Build history of the part. All positions in model axes, mm. A direction names the side the tool comes from. Round coordinates to 2 decimals unless told otherwise and drop trailing zeros. Order: outer loops, then holes, each group sorted by start corner. A loop starts at its lowest first (then second) coordinate and runs counter-clockwise, first axis right, second up. Notation, with made-up numbers: M 41,-39.5 L 72,-39.5 A33 cw 72,-2.5 Z; hole C -9,38 d7. An arc over 180 degrees is marked long. One line per item, written item: value. Start each with the question number.
Item 1: Band-saw the part on B-B, the plane x = 102. Write the cut outline in (y, z), then the cut area to 3 significant figures.
Item 2: Band-saw the part on A-A, the plane z = -15. Write the cut outline in (x, y), then the cut area to 3 significant figures.
Item 3: Band-saw the part on C-C, the plane y = 0.9. Give the number of separate pieces and of enclosed holes in the cut face, then the cut area to 3 significant figures.
Item 4: Probe L1, parallel to X at y = 2.6, z = -22.5; L2, parallel to Z at x = 81, y = 1.1; L3, parallel to X at y = 2.5, z = -5.5. List the from-to ranges inside material, lowest first.
Item 5: Band-saw the part on D-D, the plane x = 43.5. Write the cut outline in (y, z), then the cut area to 3 significant figures.
Item 6: Pin check, flat tip, straight feed: pin 1 (10 mm diameter, centred on x = -26.5, z = 28, fed in from -Y). Stop position of the tip, or through.
Item 7: Two-plate mould, pull along X, no slides. Class faces 1 (the flat face through (122.46, 1.48, -49.29)), 2 (the flat face through (2, 3, -6)), 3 (the flat face through (58.86, 1.479, -44.647)), 4 (the flat face through (-116.381, 1.479, 24.334)): +X half, -X half, draft (parallel to the pull), parting line (faces both ways), or undercut.
Item 8: Tool access for faces 5 (the flat face through (-59.14, 1.48, -44.85)), 6 (the flat face through (69.1, 1.5, 38.4)): list every direction of +Z, -Z, +X, -X, +Y, -Y with a clear straight run to the whole face (end or side of a thin tool).
```python
from build123d import *

# Parameters (mm, degrees)
SKETCH1_R           = 1.5
SKETCH1_W           = 29
SKETCH1_H           = 59.5
BOSS_EXTRUDE1_DEPTH = 3


with BuildPart() as part:
    # Sketch1 → Boss-Extrude1 (new body)
    with BuildSketch(Plane(origin=(0, 0, 0), x_dir=(1, 0, 0), z_dir=(0, 1, 0))):
        with BuildLine():
            Line((125, 46.495570398), (125, -16.504429602))
            Line((125, -16.504429602), (108, -31.946538257))
            Line((108, -31.946538257), (78, -31.946538257))
            Line((78, -31.946538257), (60, -45))
            Line((60, -45), (-60, -45))
            Line((-60, -45), (-78, -31.946538257))
            Line((-78, -31.946538257), (-108, -31.946538257))
            Line((-108, -31.946538257), (-125, -16.504429602))
            Line((-125, -16.504429602), (-125, 46.495570398))
            Line((-125, 46.495570398), (-120, 52))
            Line((-120, 52), (-69, 52))
            Line((-69, 52), (-49, 37.496153619))
            Line((-49, 37.496153619), (-38, 37.496153619))
            ThreePointArc((-38, 37.496153619), (0, 55), (38, 37.496153619))
            Line((38, 37.496153619), (49, 37.496153619))
            Line((49, 37.496153619), (69, 52))
            Line((69, 52), (120, 52))
            Line((120, 52), (125, 46.495570398))
        make_face()
        with Locations(Location((-35, 5, 0), (0, 0, 270))):
            Circle(SKETCH1_R, mode=Mode.SUBTRACT)
        with Locations(Location((-24.748737342, -19.748737342, 0), (0, 0, 270))):
            Circle(SKETCH1_R, mode=Mode.SUBTRACT)
        with Locations(Location((0, -30, 0), (0, 0, 270))):
            Circle(SKETCH1_R, mode=Mode.SUBTRACT)
        with Locations(Location((24.748737342, -19.748737342, 0), (0, 0, 270))):
            Circle(SKETCH1_R, mode=Mode.SUBTRACT)
        with Locations(Location((35, 5, 0), (0, 0, 270))):
            Circle(SKETCH1_R, mode=Mode.SUBTRACT)
        with Locations(Location((24.748737342, 29.748737342, 0), (0, 0, 270))):
            Circle(SKETCH1_R, mode=Mode.SUBTRACT)
        with Locations(Location((0, 40, 0), (0, 0, 270))):
            Circle(SKETCH1_R, mode=Mode.SUBTRACT)
        with Locations(Location((-24.748737342, 29.748737342, 0), (0, 0, 270))):
            Circle(SKETCH1_R, mode=Mode.SUBTRACT)
        with Locations((-90, 12.25)):
            Rectangle(SKETCH1_W, SKETCH1_H, mode=Mode.SUBTRACT)
        with Locations((90, 12.25)):
            Rectangle(SKETCH1_W, SKETCH1_H, mode=Mode.SUBTRACT)
    extrude(amount=BOSS_EXTRUDE1_DEPTH)


solid = part.part
```
Output:
1. outline: M 0,-52 L 3,-52 L 3,-42 L 0,-42 Z; M 0,17.5 L 3,17.5 L 3,31.95 L 0,31.95 Z
1. area: 73.3 mm²
2. outline: M -125,0 L -104.5,0 L -104.5,3 L -125,3 Z; M -75.5,0 L 75.5,0 L 75.5,3 L -75.5,3 Z; M 104.5,0 L 125,0 L 125,3 L 104.5,3 Z
2. area: 576 mm²
3. separate pieces: 1
3. enclosed holes: 10
3. area: 18,200 mm²
4. L1: x = -125 to -104.5, -75.5 to 75.5, 104.5 to 125
4. L2: z = -52 to -42, 17.5 to 31.95
4. L3: x = -125 to -104.5, -75.5 to -36.41, -33.59 to 33.59, 36.41 to 75.5, 104.5 to 125
5. outline: M 0,-37.5 L 3,-37.5 L 3,45 L 0,45 Z
5. area: 247 mm²
6. pin 1: stops at y = 0
7. face 1: +X half
7. face 2: draft
7. face 3: undercut
7. face 4: -X half
8. face 5: -Z, +Y, -Y
8. face 6: +Z, +X, +Y, -Y
